Part model, mm, in its own coordinate system. Coordinates: 2 decimals unless noted, no trailing zeros. Write each loop counter-clockwise with the first axis right and the second up, starting at its lowest first coordinate (ties: lowest second). Pieces come first, ordered by that corner, then holes. Notation, with made-up numbers: M -8,58.25 L 1,58.25 A29 cw 1,96.25 Z; hole C 40.25,-22.75 d2. An arc over 180 degrees is marked long. Use a Markdown table: item, result. Add a question column.
Q1. Slice it at B-B on y = 37.5. Write the cut outline in (x, z).
Q2. Wall check: L1, parallel to Y at x = 30, z = 0.7; L2, parallel to X at y = -0.5, z = 0.35; L3, parallel to X at y = -3, z = 1.2. Give the ranges that are in metal, low to high. Write a range as from..to.
Q3. Slice it at D-D on x = 41. Write the cut outline in (y, z), then the cut area to 3 significant figures.
Q4. Slice it at C-C on x = 8. Write the cut outline in (y, z).
Q5. Mould opens along Y. For faces 1 (the flat face through (49, 35, 1)), 2 (the cylindrical face through (84.398, 37.555, 0.986)), 3 (the cylindrical face through (82.821, 35.726, 1.014)) say: released by +Y, released by -Y, zero draft, split by the parting line, or undercut.
Q6. Pin check, flat tips, straight feed: pin 1 Ø8 at (x, y) = (66, 33) entering from -Z; pin 2 Ø1 at (x, z) = (60, 1) entering from -Y. Stop position of each tip, or through.
Q7. Slice it at A-A on z = 1.05. Write the cut outline in (x, y), then the cut area to 3 significant figures.
from build123d import *

# Parameters (mm, degrees)
BOSS_EXTRUDE1_DEPTH = 2
SKETCH4_R           = 2
CUT_EXTRUDE1_DEPTH  = 5


with BuildPart() as part:
    # Sketch1 → Boss-Extrude1 (new body)
    with BuildSketch(Plane.XY):
        with BuildLine():
            Line((9.503526384, 33.420205662), (11.898379024, 40))
            Line((11.898379024, 40), (18.900451053, 40))
            Line((18.900451053, 40), (81.898379024, 40))
            ThreePointArc((81.898379024, 40), (84.398379024, 37.5), (81.898379024, 35))
            Line((81.898379024, 35), (22.362429948, 35))
            Line((22.362429948, 35), (15.399415038, 35))
            Line((15.399415038, 35), (13.292753309, 29.212002571))
            Line((13.292753309, 29.212002571), (6.538105716, 10.653786822))
            ThreePointArc((6.538105716, 10.653786822), (-4.275251792, -11.74615776), (1.839642613, 12.363887538))
            Line((1.839642613, 12.363887538), (9.503526384, 33.420205662))
        make_face()
    extrude(amount=BOSS_EXTRUDE1_DEPTH)

    # Sketch4 → Cut-Extrude1 (cut)
    with BuildSketch(Plane.XY.offset(2)):
        with Locations((81.898379024, 37.5)):
            Circle(SKETCH4_R)
    extrude(amount=-CUT_EXTRUDE1_DEPTH, mode=Mode.SUBTRACT)


solid = part.part
Recorded:
| question | item | result |
|---|---|---|
| 1 | outline | M 10.99,0 L 79.9,0 L 79.9,2 L 10.99,2 Z; M 83.9,0 L 84.4,0 L 84.4,2 L 83.9,2 Z |
| 2 | L1 | 35..40 |
| 2 | L2 | -12.49..12.49 |
| 2 | L3 | -12.13..12.13 |
| 3 | outline | M 35,0 L 40,0 L 40,2 L 35,2 Z |
| 3 | area | 10.0 mm² |
| 4 | outline | M -9.6,0 L 9.6,0 L 9.6,2 L -9.6,2 Z; M 14.67,0 L 29.29,0 L 29.29,2 L 14.67,2 Z |
| 5 | face 1 | released by -Y |
| 5 | face 2 | split by the parting line |
| 5 | face 3 | undercut |
| 6 | pin 1 | z = 0 |
| 6 | pin 2 | y = 35 |
| 7 | outline | M 1.84,12.36 A12.5 ccw long 6.54,10.65 L 15.4,35 L 81.9,35 A2.5 ccw 81.9,40 L 11.9,40 Z; hole C 81.9,37.5 d4 |
| 7 | area | 967 mm² |
